Read the model definition and answer for the solid it produces. Units are mm, in the model's axes. A direction names the side the tool comes from. Give positions to 0.01 mm unless a question says otherwise; leave off trailing zeros. Loops run counter-clockwise (first coordinate to the right, second up) from the corner with the lowest first, then second, coordinate; pieces in that order, holes last. Notation, with made-up numbers: (62.25, -12.75) - (98.25, -12.75) arc R21 ccw to (98.25, 19.25) - close; hole circle Ø7 at (84, 33). An arc over 180 degrees is marked (long way). Write item = value, one per line. Start each with the question number.
Autodesk Inventor part; units mm, degrees
ref_plane "YZ Plane" through (0, 0, 0) normal (1, 0, 0) x (0, 1, 0)
ref_plane "XZ Plane" through (0, 0, 0) normal (0, 1, 0) x (-1, 0, 0)
ref_plane "XY Plane" through (0, 0, 0) normal (0, 0, 1) x (1, 0, 0)
sketch "草图1" plane through (0, 0, 0) normal (0, 1, 0) x (-1, 0, 0)
  circle A0 centre (0, 0) radius 6
  dimension "带轮直径" = 12
extrude "拉伸2" add sketch "草图1" along normal blind 26 draft 5
sketch "草图3" plane through (0, 0, 0) normal (0, -1, 0) x (1, 0, 0)
  circle A0 centre (0, 0) radius 10
  dimension "外径" = 20
sketch "草图4" plane through (0, 26, 0) normal (0, 1, 0) x (1, 0, 0)
  circle A0 centre (0, 0) radius 10
  dimension "d12" = 20
extrude "拉伸4" add sketch "草图3" along normal blind 2
extrude "拉伸5" add sketch "草图4" along normal blind 2
sketch "草图2" plane through (0, 0, 0) normal (0, -1, 0) x (1, 0, 0)
  circle A0 centre (0, 0) radius 5
  dimension "孔径" = 10
extrude "拉伸3" cut sketch "草图2" along normal through all both and the other way through all
equation "\"d12\" = 外径"
equation "\"d15\" = 外圆"
properties part number "带轮" material "木材(桦木)"
1. A cutting plane is placed at A-A on x = 0. Give the vertices of the cut face in (y, z).
2. Given P1, Ø5, axis at x = 5.5, y = 11, coming from the -Z side; P2, Ø3, axis at x = -1, y = 9, coming from the -Z side; P3, Ø12, axis at x = -3.5, y = 16.5, coming from the -Z side, each flat-ended and moving along its own axis, determine where each tip first touches the part or whether it passes through.
3. For a pull along Y with two mould halves and no side action, classify faces 1 (the flat face through (7, 0, 0)), 2 (the cylindrical face through (-2.17, 26.99, -9.76)), 3 (the flat face through (2, 28, -5)), 4 (the flat face through (-6, 26, -6)) as released by +Y, released by -Y, zero draft, split by the parting line, or undercut.
4. Consider line 1 along X through (y, z) = (18.5, 0); line 2 along Y through (x, z) = (4.5, 7.25); line 3 along X through (y, z) = (12.5, -1.5). Determine where each line is inside the solid, lowest interval first. Write a range as [from, to].
5. A cutting plane is placed at B-B on z = 0. Give the vertices of the cut face in (x, y), and give its area (3 significant figures).
6. A cutting plane is placed at C-C on y = 1.5. Give the vertices of the cut face in (x, z).
7. A tool of negligible diameter and unlimited length cuts with its end or side. For faces 5 (the cylindrical face through (-1.08, 12.79, -4.88)), 6 (the conical face through (7.146, 13.182, 0.315)), from which of +Z, -Z, +X, -X, +Y, -Y can it reach the whole face along a straight path? Write none if from no direction.
8. A cutting plane is placed at D-D on y = 10.25. Give the vertices of the cut face in (x, z).
Reply:
q1.outline = (-2, -10) - (0, -10) - (0, -6) - (26, -8.27) - (26, -10) - (28, -10) - (28, -5) - (-2, -5) - close; (-2, 5) - (28, 5) - (28, 10) - (26, 10) - (26, 8.27) - (0, 6) - (0, 10) - (-2, 10) - close
q2.P1 = -6.31
q2.P2 = -6.9
q2.P3 = -7.88
q3.face_1 = undercut
q3.face_2 = zero draft
q3.face_3 = released by +Y
q3.face_4 = undercut
q4.line_1 = [-7.62, -5], [5, 7.62]
q4.line_2 = [-2, 0], [26, 28]
q4.line_3 = [-6.93, -4.77], [4.77, 6.93]
q5.outline = (-10, -2) - (-5, -2) - (-5, 28) - (-10, 28) - (-10, 26) - (-8.27, 26) - (-6, 0) - (-10, 0) - close; (5, -2) - (10, -2) - (10, 0) - (6, 0) - (8.27, 26) - (10, 26) - (10, 28) - (5, 28) - close
q5.area = 151 mm^2
q6.outline = circle Ø12.26 at (0, 0); hole circle Ø10 at (0, 0)
q7.face_5 = +Y, -Y
q7.face_6 = none
q8.outline = circle Ø13.79 at (0, 0); hole circle Ø10 at (0, 0)
